Autodesk Inventor part; units mm, degrees
ref_plane "YZ Plane" through (0, 0, 0) normal (1, 0, 0) x (0, 1, 0)
ref_plane "XZ Plane" through (0, 0, 0) normal (0, 1, 0) x (-1, 0, 0)
ref_plane "XY Plane" through (0, 0, 0) normal (0, 0, 1) x (1, 0, 0)
sketch "Sketch1" plane through (0, 0, 0) normal (0, 0, 1) x (1, 0, 0)
  circle A0 centre (-74.1769, -5.2291) radius 2.1844
  circle A1 centre (-36.0455, -5.0199) radius 2.1844
  circle A2 centre (-112.2444, -5.4371) radius 2.1844
  circle A3 centre (-94.297, -37.5832) radius 2.1844
  circle A4 centre (-54.0568, 27.1251) radius 2.1844
  arc A5 (-35.4519, -11.3421) -> (-89.2225, -41.4005) centre (-28.3285, -87.2084) ccw
  arc A6 (-100.6091, -36.8907) -> (-114.967, -11.1738) centre (-125.8576, -34.1206) ccw
  arc A7 (-112.8432, 0.8846) -> (-59.1316, 30.942) centre (-120.0293, 76.745) ccw
  arc A8 (-47.7441, 26.4385) -> (-33.335, 0.7226) centre (-22.4929, 23.6923) ccw
  arc A9 (-35.4519, -11.3421) -> (-33.335, 0.7226) centre (-36.0455, -5.0199) ccw
  arc A10 (-100.6091, -36.8907) -> (-89.2225, -41.4005) centre (-94.297, -37.5832) ccw
  arc A11 (-112.8432, 0.8846) -> (-114.967, -11.1738) centre (-112.2444, -5.4371) ccw
  arc A12 (-47.7441, 26.4385) -> (-59.1316, 30.942) centre (-54.0568, 27.1251) ccw
  circle A13 centre (-61.4451, -5.159) radius 2.1844
  point P0 (-47.7441, 26.4385)
  dimension "d6" = 25.4
  dimension "d7" = 25.4
  dimension "d8" = 76.2
  dimension "d9" = 76.2
extrude "Extrusion2" add sketch "Sketch1" along normal blind 1.5875
properties part number "Side Poly"
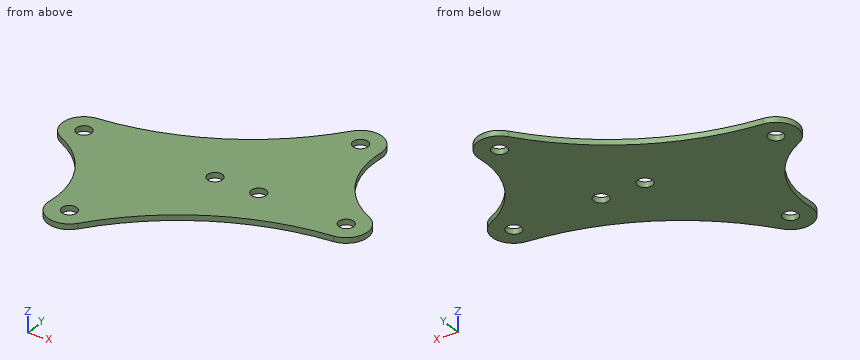
Check sheet for the modelled part. Datum: model origin and axes. Units: mm. Give positions to 0.01 mm unless a question says otherwise; leave off trailing zeros. Order: outer loops, then holes, each group sorted by start corner. A loop starts at its lowest first (then second) coordinate and runs counter-clockwise, first axis right, second up. Notation, with made-up numbers: (-16.5, 61) -> (39.5, 61) arc R19 cw to (39.5, 86) -> close; hole circle Ø6 at (-23.75, -8). An arc over 180 degrees is marked (long way). Use CSV: the item, a comma, the result in double quotes. Start each with the question number.
1) Sectioned sample at B-B, the plane z = 1.15. Record the boundary of the cut face in (x, y) (1 decimal).
2) Sectioned sample at C-C, the plane y = 7. Record the boundary of the cut face in (x, z).
3) Sectioned sample at A-A, the plane x = -62. Record the boundary of the cut face in (y, z), plus the area to 4 significant figures.
4) Go/stop test with a flat-tipped pin: P1, Ø2.5, axis at x = -36.05, y = -5.02, coming from the -Z side. Record where the tip stops, or that it passes through.
5) Material ranges on line 1 (Y direction, x = -73.5, z = 1); line 2 (Y direction, x = -55, z = 1.05); line 3 (X direction, y = -18.5, z = 1.2), recorded low to high. Write a range as from..to.
6) Sectioned sample at D-D, the plane x = -94. Record the boundary of the cut face in (y, z).
Recorded:
1,outline,"(-115, -11.2) arc R25.4 cw to (-100.6, -36.9) arc R6.3 ccw to (-89.2, -41.4) arc R76.2 cw to (-35.5, -11.3) arc R6.4 ccw to (-33.3, 0.7) arc R25.4 cw to (-47.7, 26.4) arc R6.3 ccw to (-59.1, 30.9) arc R76.2 cw to (-112.8, 0.9) arc R6.3 ccw to start; hole circle Ø4.4 at (-112.2, -5.4); hole circle Ø4.4 at (-94.3, -37.6); hole circle Ø4.4 at (-74.2, -5.2); hole circle Ø4.4 at (-61.4, -5.2); hole circle Ø4.4 at (-54.1, 27.1); hole circle Ø4.4 at (-36, -5)"
2,outline,"(-89.34, 0) -> (-41.64, 0) -> (-41.64, 1.59) -> (-89.34, 1.59) -> close"
3,outline,"(-18.85, 0) -> (-7.27, 0) -> (-7.27, 1.59) -> (-18.85, 1.59) -> close; (-3.05, 0) -> (27.36, 0) -> (27.36, 1.59) -> (-3.05, 1.59) -> close"
3,area,"66.65 mm2"
4,P1,"through"
5,line 1,"-25.84..-7.31, -3.15..16.4"
5,line 2,"-15.83..25.15, 29.1..33.4"
5,line 3,"-105.83..-61.28"
6,outline,"(-43.93, 0) -> (-39.75, 0) -> (-39.75, 1.59) -> (-43.93, 1.59) -> close; (-35.42, 0) -> (5.13, 0) -> (5.13, 1.59) -> (-35.42, 1.59) -> close"
